Read the model definition and answer for the solid it produces. Units are mm, in the model's axes. A direction names the side the tool comes from. Give positions to 0.01 mm unless a question says otherwise; leave off trailing zeros. Write each loop counter-clockwise with the first axis right and the second up, starting at its lowest first coordinate (ties: lowest second). Pieces come first, ordered by that corner, then holes. Notation, with made-up numbers: (6.5, 12) -> (31.5, 12) arc R13 ccw to (31.5, 21) -> close; hole circle Ø2 at (64, 56.25). An arc over 180 degrees is marked (long way). Use a Markdown table: item, result.
from build123d import *

# Parameters (mm, degrees)
SKETCH_1_R                           = 54
FLOOR_D108_T4P5_DEPTH                = 4.5
SKETCH_2_R                           = 54
SKETCH_2_R_2                         = 51
RIM_OD108_ID102_H24_DEPTH            = 24
SKETCH_3_R                           = 4.5
SENSOR_FIXED_POSTS_DEPTH             = 14
SKETCH_4_R                           = 2.15
M4_FIXED_MOUNT_CLEARANCE_DEPTH       = 14
SKETCH_5_R                           = 4.5
M4_FIXED_HEAD_RECESS_D8P2_T2P7_DEPTH = 2.7
SKETCH_6_W                           = 12
SKETCH_6_H                           = 11
USB_C_SIDE_OPENING_12X7_DEPTH        = 7
BASE_OUTER_ROUND_R1_R                = 1


with BuildPart() as part:
    # 草图1 → Floor_D108_T4p5 (new body)
    with BuildSketch(Plane(origin=(0, 0, 0), x_dir=(1, 0, 0), z_dir=(0, 1, 0))):
        with Locations(Location((0, 0, 0), (0, 0, 270))):
            Circle(SKETCH_1_R)
    extrude(amount=FLOOR_D108_T4P5_DEPTH)

    # 草图2 → Rim_OD108_ID102_H24 (add)
    with BuildSketch(Plane(origin=(0, 0, 0), x_dir=(1, 0, 0), z_dir=(0, 1, 0))):
        with Locations(Location((0, 0, 0), (0, 0, 270))):
            Circle(SKETCH_2_R)
        with Locations(Location((0, 0, 0), (0, 0, 270))):
            Circle(SKETCH_2_R_2, mode=Mode.SUBTRACT)
    extrude(amount=RIM_OD108_ID102_H24_DEPTH)

    # 草图3 → Sensor_fixed_posts (add)
    with BuildSketch(Plane(origin=(0, 0, 0), x_dir=(1, 0, 0), z_dir=(0, 1, 0))):
        with Locations(Location((22, 0, 0), (0, 0, 270))):
            Circle(SKETCH_3_R)
        with Locations(Location((32, 0, 0), (0, 0, 270))):
            Circle(SKETCH_3_R)
    extrude(amount=SENSOR_FIXED_POSTS_DEPTH)

    # 草图4 → M4_fixed_mount_clearance (cut)
    with BuildSketch(Plane(origin=(0, 0, 0), x_dir=(1, 0, 0), z_dir=(0, 1, 0))):
        with Locations(Location((22, 0, 0), (0, 0, 270))):
            Circle(SKETCH_4_R)
        with Locations(Location((32, 0, 0), (0, 0, 270))):
            Circle(SKETCH_4_R)
    extrude(amount=M4_FIXED_MOUNT_CLEARANCE_DEPTH, mode=Mode.SUBTRACT)

    # 草图5 → M4_fixed_head_recess_D8p2_T2p7 (cut)
    with BuildSketch(Plane(origin=(0, 0, 0), x_dir=(1, 0, 0), z_dir=(0, 1, 0))):
        with Locations(Location((22, 0, 0), (0, 0, 270))):
            Circle(SKETCH_5_R)
        with Locations(Location((32, 0, 0), (0, 0, 270))):
            Circle(SKETCH_5_R)
    extrude(amount=M4_FIXED_HEAD_RECESS_D8P2_T2P7_DEPTH, mode=Mode.SUBTRACT)

    # 草图6 → USB_C_side_opening_12x7 (cut)
    with BuildSketch(Plane(origin=(0, 8, 0), x_dir=(1, 0, 0), z_dir=(0, 1, 0))):
        with Locations((0, 54.5)):
            Rectangle(SKETCH_6_W, SKETCH_6_H)
    extrude(amount=USB_C_SIDE_OPENING_12X7_DEPTH, mode=Mode.SUBTRACT)

    # Base_outer_round_R1
    base_outer_round_r1_edges = [part.edges().sort_by_distance(p)[0] for p in [
        (0, 24, -54),
    ]]
    fillet(base_outer_round_r1_edges, radius=BASE_OUTER_ROUND_R1_R)


solid = part.part
Item 1: For a pull along Z with two mould halves and no side action, classify faces 4 (the face through (-20.682, 11.339, 49.882)), 5 (the face through (0, 15, -52)), 6 (the face through (33.81, 8.27, 1.16)) as +Z half, -Z half, draft (parallel to the pull), parting line (faces both ways), or undercut.
Return value:
| item | result |
|---|---|
| face 4 | parting line |
| face 5 | draft |
| face 6 | undercut |
Item 2: Each of these flat-tipped pins is pushed along its axis until it touches: P1, Ø2, axis at y = 12.5, z = -7.5, coming from the +X side; P2, Ø7, axis at x = 30.5, z = 1.5, coming from the -Y side; P3, Ø2.5, axis at x = 21, z = -1, coming from the +Y side; P4, Ø1, axis at x = -9.5, z = 17, coming from the +Y side. Where does it stop, or does it pass through?
Return value:
| item | result |
|---|---|
| P1 | x = 53.61 |
| P2 | y = 0 |
| P3 | y = 14 |
| P4 | y = 4.5 |
Item 3: A cutting plane is placed at B-B (z = 0). Count the separate pieces of the cut face and the enclosed holes in it, then the cut area to 3 significant figures.
Return value:
| item | result |
|---|---|
| separate pieces | 3 |
| enclosed holes | 0 |
| area | 628 mm^2 |
Item 4: A tool of negligible diameter and unlimited length cuts with its end or side. For faces 1 (the face through (1, 4.5, -1)), 2 (the face through (26.46, 1.33, -0.59)), 3 (the face through (6, 11, -52)), from which of +Z, -Z, +X, -X, +Y, -Y can it reach the whole face along a straight path? Write none if from no direction.
Return value:
| item | result |
|---|---|
| face 1 | +Y |
| face 2 | -Y |
| face 3 | -Z |
Item 5: Straight lines are drawn through the part: line 1 along X through (y, z) = (1.55, 0); line 2 along X through (y, z) = (10.75, 0); line 3 along Z through (x, y) = (32, 6.25). For each, find the intervals that lie inside material, in ascending order. Write a range as [from, to].
Return value:
| item | result |
|---|---|
| line 1 | [-54, 17.5], [26.5, 27.5], [36.5, 54] |
| line 2 | [-54, -51], [17.5, 19.85], [24.15, 26.5], [27.5, 29.85], [34.15, 36.5], [51, 54] |
| line 3 | [-43.5, -39.71], [-4.5, -2.15], [2.15, 4.5], [39.71, 43.5] |
Item 6: A cutting plane is placed at C-C (y = 16.75). Give the vertices of the cut face in (x, z).
Return value:
| item | result |
|---|---|
| outline | circle Ø108 at (0, 0); hole circle Ø102 at (0, 0) |
Item 7: A cutting plane is placed at A-A (x = 0). Give the vertices of the cut face in (y, z), then the cut area to 3 significant figures.
Return value:
| item | result |
|---|---|
| outline | (0, -54) -> (8, -54) -> (8, -51) -> (4.5, -51) -> (4.5, 51) -> (24, 51) -> (24, 53) arc R1 ccw to (23, 54) -> (0, 54) -> close; (15, -54) -> (23, -54) arc R1 ccw to (24, -53) -> (24, -51) -> (15, -51) -> close |
| area | 582 mm^2 |
